```python
from build123d import *

# Parameters (mm, degrees)
CROQUIS2_R              = 1.5
SALIENTE_EXTRUIR1_DEPTH = 1
ESCALA1_SCALE           = 7


with BuildPart() as part:
    # Croquis2 → Saliente-Extruir1 (new body)
    with BuildSketch(Plane.XY):
        with BuildLine():
            ThreePointArc((3.5, 47.5), (0, 51), (-3.5, 47.5))
            ThreePointArc((-3.5, 47.5), (-3.029104107, 25.977421026), (-4.5, 4.5))
            ThreePointArc((-4.5, 4.5), (0, 0), (4.5, 4.5))
            ThreePointArc((4.5, 4.5), (3.029104107, 25.977421026), (3.5, 47.5))
        make_face()
        with Locations((0, 47.5)):
            Circle(CROQUIS2_R, mode=Mode.SUBTRACT)
        with Locations((0, 4.5)):
            Circle(CROQUIS2_R, mode=Mode.SUBTRACT)
    extrude(amount=SALIENTE_EXTRUIR1_DEPTH)


with BuildPart() as part_1:
    # Escala1: scaled about (0, 24.124187823, 0.5)
    add(part.part.scale(ESCALA1_SCALE).moved(Location((0, -144.745126938, -3))))


solid = part_1.part
```
Geometry: final body of the model. Coordinates: model frame, mm. Round coordinates to 2 decimals unless told otherwise and drop trailing zeros. Write each loop counter-clockwise with the first axis right and the second up, starting at its lowest first coordinate (ties: lowest second). Pieces come first, ordered by that corner, then holes.
Item 1: Section query B-B (z = 1.25). Return loops of the section in (x, y), plus the area to 3 significant figures.
Item 2: Section query C-C (y = 42). Return loops of the section in (x, z), plus the area to 3 significant figures.
Item 3: Pin query (flat end, axial travel): P1, Ø1.5, axis at x = -19.5, z = 2, coming from the +Y side; P2, Ø1, axis at x = 18.5, z = 3, coming from the +Y side; P3, Ø4, axis at x = -14.5, z = 2, coming from the +Y side. Return the tip coordinate at first contact, or that it passes through.
Item 4: Mould query, pull axis X, two halves, no side actions, for faces 1 (the face through (0, 36, 4)), 2 (the face through (-21.156, 39.207, 0.451)), 3 (the face through (4.85, -122.56, 0.45)). Classes: +X half, -X half, draft (parallel to the pull), parting line (faces both ways), or undercut.
Item 5: Section query A-A (x = 0). Return loops of the section in (y, z).
Item 6: Section query D-D (x = 28). Return loops of the section in (y, z).
Item 7: Material intervals for L1, parallel to Y at x = 1, z = 3.5; L2, parallel to Y at x = 0, z = 1.25; L3, parallel to X at y = 67.5, z = 2.75, sorted ascending.
Completed:
1. outline: (-31.5, -113.25) arc R31.5 ccw to (31.5, -113.25) arc R1670.22 cw to (24.5, 187.75) arc R24.5 ccw to (-24.5, 187.75) arc R1670.22 cw to start; hole circle Ø21 at (0, -113.25); hole circle Ø21 at (0, 187.75)
1. area: 15,900 mm2
2. outline: (-21.1, -3) - (21.1, -3) - (21.1, 4) - (-21.1, 4) - close
2. area: 295 mm2
3. P1: stops at y = 203.52
3. P2: stops at y = 204.38
3. P3: stops at y = 208.83
4. face 1: draft
4. face 2: -X half
4. face 3: undercut
5. outline: (-144.75, -3) - (-123.75, -3) - (-123.75, 4) - (-144.75, 4) - close; (-102.75, -3) - (177.25, -3) - (177.25, 4) - (-102.75, 4) - close; (198.25, -3) - (212.25, -3) - (212.25, 4) - (198.25, 4) - close
6. outline: (-127.68, -3) - (-79.5, -3) - (-79.5, 4) - (-127.68, 4) - close
7. L1: y = -144.73 to -123.7, -102.79 to 177.3, 198.21 to 212.23
7. L2: y = -144.75 to -123.75, -102.75 to 177.25, 198.25 to 212.25
7. L3: x = -20.77 to 20.77
